from build123d import *

# Parameters (mm, degrees)
SKETCH1_R                  = 4.7625
BOSS_EXTRUDE1_DEPTH        = 114.3
F_10_32_TAPPED_HOLE1_D     = 4.0386
F_10_32_TAPPED_HOLE1_DEPTH = 11.938


with BuildPart() as part:
    # Sketch1 → Boss-Extrude1 (new body, symmetric)
    with BuildSketch(Plane(origin=(0, 0, 0), x_dir=(0, 0, -1), z_dir=(1, 0, 0))):
        Circle(SKETCH1_R)
    extrude(amount=BOSS_EXTRUDE1_DEPTH, both=True)

    # #10-32 Tapped Hole1
    with Locations(Plane.ZY.offset(114.3)):
        with Locations((0, 0)):
            f_10_32_tapped_hole1 = Hole(F_10_32_TAPPED_HOLE1_D / 2, depth=F_10_32_TAPPED_HOLE1_DEPTH)

    # Mirror1: #10-32 Tapped Hole1 across plane
    add(f_10_32_tapped_hole1.mirror(Plane(origin=(0, 0, 0), x_dir=(0, 0, 1), z_dir=(1, 0, 0))), mode=Mode.SUBTRACT)


solid = part.part
Can you work these out from the model? Positions are in its coordinate system, mm. A direction names the side the tool comes from. Round coordinates to 2 decimals unless told otherwise and drop trailing zeros. Write each loop counter-clockwise with the first axis right and the second up, starting at its lowest first coordinate (ties: lowest second). Pieces come first, ordered by that corner, then holes. Notation, with made-up numbers: (61.5, -7.5) -> (93.5, -7.5) arc R11 ccw to (93.5, 2.5) -> close; hole circle Ø10 at (88.25, 38). An arc over 180 degrees is marked (long way). One line per question, with ' | ' between items. Start each with the question number.
1) If we mould it in two halves opening along Y, with no side actions, what happens to faces 1 (the flat face through (114.3, -1, -2)), 2 (the cylindrical face through (108.247, 0.607, -1.926)), 3 (the flat face through (-102.362, 0, 0)), 4 (the cylindrical face through (1.6, -2.9, 3.78))? For each: released by +Y, released by -Y, zero draft, split by the parting line, or undercut.
2) I need wall thicknesses on line 1 (Y direction, x = 107.5, z = 0); line 2 (X direction, y = 1.5, z = 0.5); line 3 (Y direction, x = -23.5, z = 0.5). Which ranges of each line are inside material? Lowest first, please. Write a range as [from, to].
3) Suppose I cut it at A-A on z = 0. Write out the boundary of the cut face in (x, y), then the cut area to 3 significant figures.
4) Suppose I cut it at C-C on x = -50.5. Write out the boundary of the cut face in (y, z) (1 decimal), then the cut area to 3 significant figures.
5) I'm going to push flat-ended pins straight in: P1, Ø2.5, axis at y = 0, z = 0, coming from the -X side; P2, Ø1.5, axis at x = 13.5, z = 2, coming from the -Y side; P3, Ø1, axis at x = -16.5, y = 2.5, coming from the -Z side. Where does each tip first touch, or does it pass through?
6) On a 3-axis mill with a long thin cutter (end or side, diameter ignored), from which of +Z, -Z, +X, -X, +Y, -Y can I reach the whole of each face in a straight line? I mean faces 5 (the flat face through (102.362, 0, 0)), 6 (the flat face through (-114.3, -1, -2)), 7 (the cylindrical face through (-108.247, 0.607, -1.926)). Say none if no direction works.
Return value:
1) face 1: zero draft | face 2: undercut | face 3: undercut | face 4: split by the parting line
2) line 1: y = [-4.76, -2.02], [2.02, 4.76] | line 2: x = [-102.36, 102.36] | line 3: y = [-4.74, 4.74]
3) outline: (-114.3, -4.76) -> (114.3, -4.76) -> (114.3, -2.02) -> (102.36, -2.02) -> (102.36, 2.02) -> (114.3, 2.02) -> (114.3, 4.76) -> (-114.3, 4.76) -> (-114.3, 2.02) -> (-102.36, 2.02) -> (-102.36, -2.02) -> (-114.3, -2.02) -> close | area: 2,080 mm2
4) outline: circle Ø9.5 at (0, 0) | area: 71.3 mm2
5) P1: stops at x = -102.36 | P2: stops at y = -4.6 | P3: stops at z = -4.32
6) face 5: +X | face 6: +Z, -Z, -X, +Y, -Y | face 7: -X
